from build123d import *

# Parameters (mm, degrees)
SKETCH1_R           = 2
BOSS_EXTRUDE1_DEPTH = 2.5
SKETCH2_R           = 1
BOSS_EXTRUDE2_DEPTH = 10
CUT_EXTRUDE3_DEPTH  = 0.5


with BuildPart() as part:
    # Sketch1 → Boss-Extrude1 (new body)
    with BuildSketch(Plane(origin=(0, 0, 0), x_dir=(1, 0, 0), z_dir=(0, 1, 0))):
        Circle(SKETCH1_R)
    extrude(amount=BOSS_EXTRUDE1_DEPTH)

    # Sketch2 → Boss-Extrude2 (add)
    with BuildSketch(Plane(origin=(0, 2.5, 0), x_dir=(1, 0, 0), z_dir=(0, 1, 0))):
        Circle(SKETCH2_R)
    extrude(amount=BOSS_EXTRUDE2_DEPTH)

    # Sketch3 → Cut-Extrude3 (cut)
    with BuildSketch(Plane.XZ):
        with BuildLine():
            Line((-1.732050808, 1), (0, 2))
            ThreePointArc((0, 2), (-1, 1.732050808), (-1.732050808, 1))
        make_face()
        with BuildLine():
            Line((-1.732050808, -1), (-1.732050808, 1))
            ThreePointArc((-1.732050808, 1), (-2, 0), (-1.732050808, -1))
        make_face()
        with BuildLine():
            Line((0, -2), (-1.732050808, -1))
            ThreePointArc((-1.732050808, -1), (-1, -1.732050808), (0, -2))
        make_face()
        with BuildLine():
            ThreePointArc((0, -2), (1, -1.732050808), (1.732050808, -1))
            Line((1.732050808, -1), (0, -2))
        make_face()
        with BuildLine():
            ThreePointArc((2, 0), (1.931851653, 0.51763809), (1.732050808, 1))
            Line((1.732050808, 1), (1.732050808, -1))
            ThreePointArc((1.732050808, -1), (1.931851653, -0.51763809), (2, 0))
        make_face()
        with BuildLine():
            ThreePointArc((1.732050808, 1), (1, 1.732050808), (0, 2))
            Line((0, 2), (1.732050808, 1))
        make_face()
    extrude(amount=-CUT_EXTRUDE3_DEPTH, mode=Mode.SUBTRACT)


solid = part.part
Work out the finished part from the listing and answer in its coordinate system (mm). A direction names the side the tool comes from. Round coordinates to 2 decimals unless told otherwise and drop trailing zeros. Order: outer loops, then holes, each group sorted by start corner. A loop starts at its lowest first (then second) coordinate and runs counter-clockwise, first axis right, second up. Notation, with made-up numbers: M -24,57.5 L 9,57.5 A23 cw 9,87.5 Z; hole C 23.5,-27.5 d2. An arc over 180 degrees is marked long. One line per item, written item: value.
Q1. Straight lines are drawn through the part: line 1 (Y direction, x = -1.45, z = -0.15); line 2 (Y direction, x = 1.8, z = 0.65); line 3 (X direction, y = 6.5, z = 0.3). For each, find the intervals that lie inside material, in ascending order.
Derived:
line 1: 0 to 2.5
line 2: 0.5 to 2.5
line 3: -0.95 to 0.95
Q2. Find section B-B on x = 1.5. Write down the section's boundary in (y, z), then the cut area to 3 significant figures.
Derived:
outline: M 0,-1.13 L 0.5,-1.13 L 0.5,-1.32 L 2.5,-1.32 L 2.5,1.32 L 0.5,1.32 L 0.5,1.13 L 0,1.13 Z
area: 6.43 mm²
Q3. Find section D-D on x = -0.25. Write down the section's boundary in (y, z).
Derived:
outline: M 0,-1.86 L 0.5,-1.86 L 0.5,-1.98 L 2.5,-1.98 L 2.5,-0.97 L 12.5,-0.97 L 12.5,0.97 L 2.5,0.97 L 2.5,1.98 L 0.5,1.98 L 0.5,1.86 L 0,1.86 Z
Q4. For faces 1 (the face through (-0.88, 0.25, 1.49)), 2 (the face through (-0.85, 0.25, -1.51)), 3 (the face through (0.88, 0.25, -1.49)), determine the directions among +Z, -Z, +X, -X, +Y, -Y from which every point of the face is accessible in a straight line to the end or side of a thin tool.
Derived:
face 1: +Z, -X, -Y
face 2: -Z, -X, -Y
face 3: -Z, +X, -Y
Q5. A flat-ended cylindrical pin translates along its axis: pin 1 (1 mm diameter, centred on y = 8, z = 0, fed in from +X). Find the tip coordinate at first contact, or state that the pin passes through.
Derived:
pin 1: x = 1
Q6. Find section A-A on z = 0. Write down the section's boundary in (x, y).
Derived:
outline: M -2,0.5 L -1.73,0.5 L -1.73,0 L 1.73,0 L 1.73,0.5 L 2,0.5 L 2,2.5 L 1,2.5 L 1,12.5 L -1,12.5 L -1,2.5 L -2,2.5 Z
Q7. Find section C-C on y = 5.5. Write down the section's boundary in (x, z).
Derived:
outline: C 0,0 d2
